Could you check a few things on this model? Use its own coordinates, in mm. A direction names the side the tool comes from. Round coordinates to 2 decimals unless told otherwise and drop trailing zeros. Loops run counter-clockwise (first coordinate to the right, second up) from the corner with the lowest first, then second, coordinate; pieces in that order, holes last. Notation, with made-up numbers: (65.5, -38) -> (122.5, -38) arc R23 ccw to (122.5, -11) -> close; hole circle Ø5 at (-20.5, 24.25). An arc over 180 degrees is marked (long way). Put each result on its own line as item: value. Start each with the question number.
1. I'm going to push flat-ended pins straight in: P1, Ø5.5, axis at y = 12.7, z = -12.7, coming from the -X side; P2, Ø5.5, axis at y = 10, z = -12, coming from the +X side (3 decimals); P3, Ø15, axis at x = 12.7, y = 12.7, coming from the +Z side (3 decimals); P4, Ø8.5, axis at x = 11.5, y = 16.5, coming from the -Z side. Where does each tip first touch, or does it pass through?
2. Imagine slicing it at D-D, the plane z = -12. Please give me the cut outline in (x, y) (1 decimal), and give its area (3 significant figures).
3. Imagine slicing it at B-B, the plane z = -23.5. Please give me the cut outline in (x, y).
4. If we mould it in two halves opening along X, with no side actions, what happens to faces 6 (the flat face through (25.4, 4, -18)), 7 (the cylindrical face through (19.9, 15.5, -11.2)), 8 (the cylindrical face through (11.2, 15.5, -5.5))? For each: pulls with the +X half, pulls with the -X half, needs draft (parallel to the pull), parting line crosses it, or undercut.
5. Imagine slicing it at C-C, the plane x = 21.75. Please give me the cut outline in (y, z) (3 decimals), and give its area (3 significant figures).
6. Which directions (+Z, -Z, +X, -X, +Y, -Y) give clear straight access to the entire face, cutting with the end or side of a thin tool? Please do faces 1 (the flat face through (9, 17, -7.938)), 2 (the cylindrical face through (5.68, 1.57, -6.26)), 3 (the flat face through (10, 15, -3.175)), 4 (the flat face through (18, 4, 0)), 5 (the flat face through (22.225, 13, -9)).
7. I need wall thicknesses on line 1 (X direction, y = 12.7, z = -1.7) (3 decimals); line 2 (X direction, y = 5.6, z = -12.7) (3 decimals); line 3 (Z direction, x = 23.1, y = 12.7) (3 decimals). Which ranges of each line are inside material? Lowest first, please. Write a range as [from, to].
8. Imagine slicing it at A-A, the plane y = 15.5. Please give me the cut outline in (x, z) (1 decimal).
Autodesk Inventor part; units mm, degrees
ref_plane "YZ Plane" through (0, 0, 0) normal (1, 0, 0) x (0, 1, 0)
ref_plane "XZ Plane" through (0, 0, 0) normal (0, 1, 0) x (-1, 0, 0)
ref_plane "XY Plane" through (0, 0, 0) normal (0, 0, 1) x (1, 0, 0)
sketch "Sketch1" plane through (0, 0, 0) normal (0, 1, 0) x (-1, 0, 0)
  line L0 (0, 0) -> (-25.4, 0)
  line L1 (-25.4, 0) -> (-25.4, -25.4)
  line L2 (-25.4, -25.4) -> (0, -25.4)
  line L3 (0, -25.4) -> (0, 0)
  line L4 (0, 0) -> (-25.4, -25.4) construction
  line L5 (-25.4, 0) -> (0, -25.4) construction
  circle A0 centre (-12.7, -12.7) radius 9.525
  dimension "d0" = 25.4
  dimension "d1" = 25.4
  dimension "d3" = 19.05
extrude "Extrusion1" add sketch "Sketch1" along normal blind 3.175
sketch "Sketch2" plane through (0, 3.175, 0) normal (0, 1, 0) x (1, 0, 0)
  line L0 (25.4, 25.4) -> (0, 25.4)
  line L1 (0, 0) -> (25.4, 0)
  line L2 (25.4, 0) -> (25.4, 25.4)
  line L3 (25.4, 25.4) -> (0, 25.4)
  line L4 (0, 25.4) -> (0, 0)
  line L5 (0, 25.4) -> (0, 0) construction
  line L6 (0, 0) -> (25.4, 25.4) construction
  line L7 (0, 25.4) -> (25.4, 0) construction
  circle A0 centre (12.7, 12.7) radius 3.175
  dimension "d39" = 6.35
extrude "Extrusion2" add sketch "Sketch2" along normal blind 4.7625
sketch "Sketch4" plane through (0, 0, 0) normal (0, 0, 1) x (1, 0, 0)
  line L0 (0, 0) -> (0, 7.9375)
  line L1 (0, 0) -> (25.4, 0)
  line L2 (25.4, 0) -> (25.4, 25.4)
  line L3 (25.4, 25.4) -> (0, 25.4)
  line L4 (0, 25.4) -> (0, 0)
  line L5 (0, 25.4) -> (25.4, 0) construction
  line L6 (25.4, 25.4) -> (0, 0) construction
  circle A0 centre (12.7, 12.7) radius 9.525
  dimension "d13" = 25.4
  dimension "d14" = 25.4
  dimension "d15" = 19.05
extrude "Extrusion4" add sketch "Sketch4" against normal blind 3.175
sketch "Sketch5" plane through (0, 0, 0) normal (0, 0, 1) x (1, 0, 0)
  line L0 (0, 0) -> (0, 25.4) construction
  line L1 (0, 0) -> (25.4, 0) construction
  line L2 (0, 25.4) -> (25.4, 0) construction
  line L3 (0, 25.4) -> (25.4, 25.4) construction
  line L4 (25.4, 0) -> (25.4, 25.4) construction
  line L5 (0, 0) -> (0, 7.9375) construction
  line L6 (25.4, 25.4) -> (0, 0) construction
  circle A0 centre (12.7, 12.7) radius 9.525
  dimension "d18" = 19.05
extrude "Extrusion5" cut sketch "Sketch5" against normal blind 3.175
sketch "Sketch6" plane through (0, 0, -3.175) normal (0, 0, -1) x (-1, 0, 0)
  line L0 (-25.4, 0) -> (-25.4, 25.4)
  line L1 (-25.4, 25.4) -> (0, 25.4)
  line L2 (0, 25.4) -> (0, 0)
  line L3 (0, 0) -> (-25.4, 0)
  line L4 (-25.4, 0) -> (-25.4, 25.4)
  line L5 (0, 0) -> (0, 25.4) construction
  line L6 (-25.4, 25.4) -> (0, 0) construction
  line L7 (0, 0) -> (0, 25.4) construction
  line L8 (0, 25.4) -> (-25.4, 0) construction
  circle A0 centre (-12.7, 12.7) radius 3.175
  dimension "d40" = 6.35
extrude "Extrusion6" add sketch "Sketch6" along normal blind 4.7625
sketch "Sketch7" plane through (25.4, 0, 0) normal (1, 0, 0) x (0, 0, -1)
  line L0 (0, 25.4) -> (7.9375, 25.4)
  line L1 (25.4, 0) -> (25.4, 7.9375)
  line L2 (0, 25.4) -> (25.4, 25.4)
  line L3 (25.4, 25.4) -> (25.4, 0)
  line L4 (25.4, 0) -> (0, 0)
  line L5 (0, 0) -> (0, 25.4)
  line L6 (0, 25.4) -> (25.4, 0) construction
  line L7 (25.4, 25.4) -> (0, 0) construction
  circle A0 centre (12.7, 12.7) radius 9.525
  dimension "d24" = 19.05
extrude "Extrusion7" add sketch "Sketch7" against normal blind 3.175
sketch "Sketch8" plane through (25.4, 0, 0) normal (1, 0, 0) x (0, 0, -1)
  line L0 (0, 0) -> (0, 25.4) construction
  line L1 (0, 0) -> (25.4, 0) construction
  line L2 (0, 25.4) -> (25.4, 0) construction
  line L3 (25.4, 0) -> (25.4, 25.4) construction
  line L4 (25.4, 25.4) -> (0, 0) construction
  circle A0 centre (12.7, 12.7) radius 9.525
  dimension "d27" = 19.05
extrude "Extrusion8" cut sketch "Sketch8" against normal blind 3.175
sketch "Sketch9" plane through (22.225, 0, 0) normal (-1, 0, 0) x (0, 0, 1)
  line L0 (-25.4, 25.4) -> (-25.4, 7.9375)
  line L1 (-25.4, 25.4) -> (0, 25.4)
  line L2 (0, 25.4) -> (0, 0)
  line L3 (0, 0) -> (-25.4, 0)
  line L4 (-25.4, 0) -> (-25.4, 25.4)
  line L5 (-25.4, 0) -> (0, 0) construction
  line L6 (-25.4, 25.4) -> (0, 0) construction
  line L7 (0, 0) -> (0, 25.4) construction
  line L8 (0, 25.4) -> (-25.4, 0) construction
  circle A0 centre (-12.7, 12.7) radius 3.175
  dimension "d41" = 6.35
extrude "Extrusion9" add sketch "Sketch9" along normal blind 4.7625
sketch "Sketch10" plane through (0, 0, 0) normal (0, -1, 0) x (1, 0, 0)
  line L0 (0, -25.4) -> (0, -7.9375)
  line L1 (25.4, 0) -> (0, 0)
  line L2 (0, -25.4) -> (25.4, -25.4)
  line L3 (25.4, -25.4) -> (25.4, 0)
  line L4 (25.4, 0) -> (0, 0)
  line L5 (0, 0) -> (0, -25.4)
  line L6 (17.4625, -25.4) -> (0, -25.4) construction
  line L7 (25.4, 0) -> (25.4, -25.4) construction
  line L8 (0, -25.4) -> (25.4, 0) construction
  line L9 (25.4, 0) -> (0, 0) construction
  line L10 (0, -25.4) -> (0, 0) construction
  line L11 (0, 0) -> (25.4, -25.4) construction
  circle A0 centre (12.7, -12.7) radius 9.525
  dimension "d33" = 19.05
extrude "Extrusion10" cut sketch "Sketch10" against normal blind 3.175 contours A0
sketch "Sketch11" plane through (0, 0, 0) normal (0, 0, 1) x (1, 0, 0)
  line L0 (0, 7.9375) -> (0, 25.4) construction
  line L1 (25.4, 0) -> (25.4, 25.4) construction
  line L2 (0, 25.4) -> (25.4, 0) construction
  line L3 (25.4, 0) -> (25.4, 25.4) construction
  line L4 (25.4, 25.4) -> (0, 0) construction
  circle A0 centre (12.7, 12.7) radius 9.525
  dimension "d36" = 19.05
extrude "Extrusion11" cut sketch "Sketch11" against normal blind 3.175
properties part number "MountingBracket_2"
Entries:
1. P1: through
1. P2: x = 22.225
1. P3: z = -3.175
1. P4: z = -7.94
2. outline: (0, 0) -> (3.2, 0) -> (3.2, 3.2) -> (9.6, 3.2) -> (9.6, 7.9) -> (0, 7.9) -> close; (15.8, 3.2) -> (22.2, 3.2) -> (22.2, 0) -> (25.4, 0) -> (25.4, 3.2) -> (22.2, 3.2) -> (22.2, 9.6) -> (17.5, 9.6) -> (17.5, 7.9) -> (15.8, 7.9) -> close; (17.5, 15.8) -> (22.2, 15.8) -> (22.2, 22.2) -> (25.4, 22.2) -> (25.4, 25.4) -> (17.5, 25.4) -> close
2. area: 161 mm^2
3. outline: (0, 0) -> (25.4, 0) -> (25.4, 25.4) -> (17.46, 25.4) -> (17.46, 7.94) -> (0, 7.94) -> close
4. face 6: pulls with the +X half
4. face 7: needs draft
4. face 8: undercut
5. outline: (0, -25.4) -> (25.4, -25.4) -> (25.4, 0) -> (15.67, 0) -> (15.67, -3.175) -> (9.73, -3.175) -> (9.73, 0) -> (0, 0) -> (0, -9.73) -> (3.175, -9.73) -> (3.175, -15.67) -> (0, -15.67) -> close; hole circle Ø6.35 at (12.7, -12.7)
5. area: 576 mm^2
6. face 1: -Z, -X, +Y
6. face 2: -Y
6. face 3: +Z
6. face 4: +Z, +X, -X, +Y, -Y
6. face 5: +X
7. line 1: [0, 3.175], [22.225, 25.4]
7. line 2: [0, 9.525], [15.875, 22.225]
7. line 3: [-25.4, -22.225], [-3.175, 0]
8. outline: (0, -7.9) -> (11.2, -7.9) -> (11.2, -3.2) -> (3.6, -3.2) -> (3.6, 0) -> (0, 0) -> close; (14.2, -7.9) -> (17.5, -7.9) -> (17.5, -11.2) -> (22.2, -11.2) -> (22.2, -3.6) -> (25.4, -3.6) -> (25.4, 0) -> (21.8, 0) -> (21.8, -3.2) -> (14.2, -3.2) -> close; (17.5, -25.4) -> (25.4, -25.4) -> (25.4, -21.8) -> (22.2, -21.8) -> (22.2, -14.2) -> (17.5, -14.2) -> close
